Job drawing, mm, ordinate dimensions from the low corner. One solid piece. Round coordinates to 2 decimals unless told otherwise and drop trailing zeros. Loops run counter-clockwise (first coordinate to the right, second up) from the corner with the lowest first, then second, coordinate; pieces in that order, holes last. Notation, with made-up numbers: M 60.25,-36 L 106.25,-36 A18 cw 106.25,-24 Z; hole C 4.25,82.5 d1. An arc over 180 degrees is marked long. Use a Markdown table: item, result. Add a question column.
(1) Band-saw the part on A-A, the plane x = 85. Write the cut outline in (y, z), and give its area (3 significant figures).
(2) Wall check: L1, parallel to Y at x = 80.05, z = 1.2; L2, parallel to X at y = 89, z = 2.5. Give the ranges that are in metal, low to high.
(3) Flat gauge pin, fed straight in: P1, Ø2.5, axis at x = 89.95, y = 80.05, coming from the +Z side. Where does the tip first touch, or does it go through?
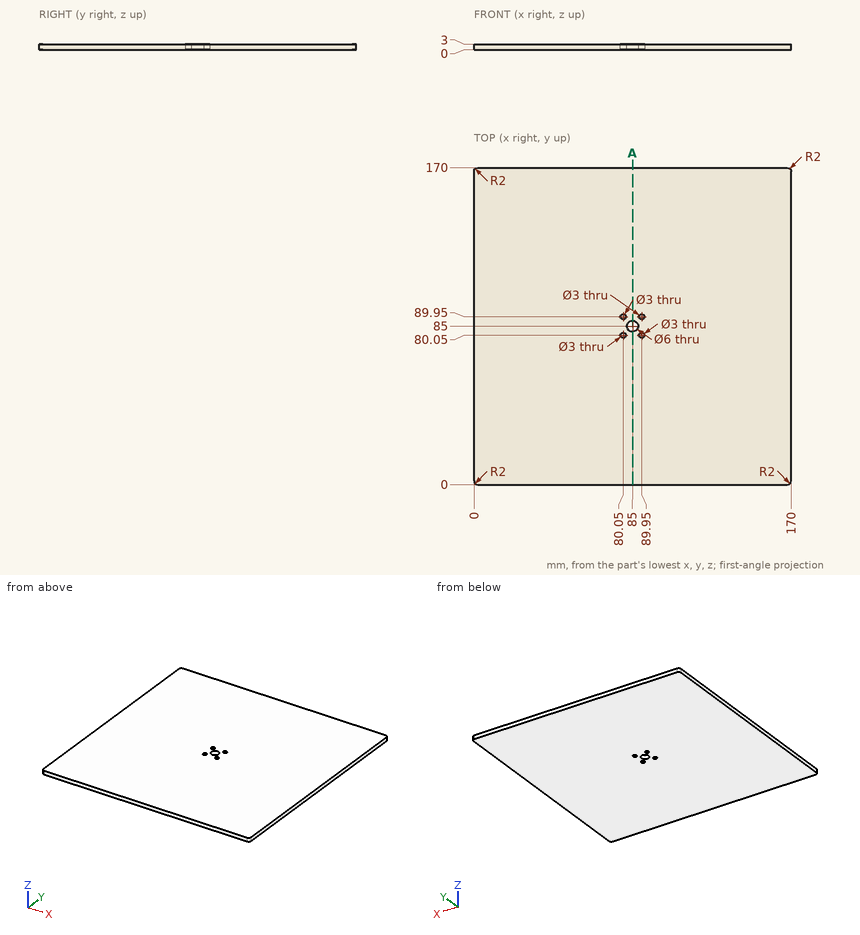
Return value:
| question | item | result |
|---|---|---|
| 1 | outline | M 0,0 L 82,0 L 82,3 L 0,3 Z; M 88,0 L 170,0 L 170,3 L 88,3 Z |
| 1 | area | 492 mm^2 |
| 2 | L1 | 0 to 78.55, 81.55 to 88.45, 91.45 to 170 |
| 2 | L2 | 0 to 78.89, 81.21 to 88.79, 91.11 to 170 |
| 3 | P1 | through |
